```python
from build123d import *

# Parameters (mm, degrees)
SKETCH1_W           = 60
SKETCH1_H           = 60
BOSS_EXTRUDE1_DEPTH = 6
SKETCH2_R           = 1.15
CUT_EXTRUDE1_DEPTH  = 43.848570571
SKETCH3_R           = 1.15
CUT_EXTRUDE2_DEPTH  = 4
CUT_EXTRUDE3_DEPTH  = 3
SKETCH5_R           = 1.15
CUT_EXTRUDE4_DEPTH  = 43.532340636


with BuildPart() as part:
    # Sketch1 → Boss-Extrude1 (new body)
    with BuildSketch(Plane.XY):
        Rectangle(SKETCH1_W, SKETCH1_H)
    extrude(amount=BOSS_EXTRUDE1_DEPTH)

    # Sketch2 → Cut-Extrude1 (cut, through all)
    with BuildSketch(Plane.XY.offset(6)):
        with BuildLine():
            ThreePointArc((-25, 26.15), (-26.15, 25), (-25, 23.85))
            Line((-25, 23.85), (-25, 26.15))
        make_face()
        with BuildLine():
            Line((-25, 26.15), (-25, 23.85))
            ThreePointArc((-25, 23.85), (-24.186827202, 24.186827202), (-23.85, 25))
            ThreePointArc((-23.85, 25), (-24.186827202, 25.813172798), (-25, 26.15))
        make_face()
        with Locations((25, 25)):
            Circle(SKETCH2_R)
        with Locations((25, -25)):
            Circle(SKETCH2_R)
        with Locations((-25, -25)):
            Circle(SKETCH2_R)
    extrude(amount=-CUT_EXTRUDE1_DEPTH, mode=Mode.SUBTRACT)

    # Sketch3 → Cut-Extrude2 (cut)
    # profile 1 of 4: a face of its own
    with BuildSketch(Plane.XY.offset(6)):
        Polygon((-26.212435565, 22.9), (-23.787564435, 22.9), (-22.575128869, 25), (-23.787564435, 27.1), (-26.212435565, 27.1), (-27.424871131, 25), align=None)
        with Locations((-25, 25)):
            Circle(SKETCH3_R, mode=Mode.SUBTRACT)
    # profile 2 of 4: a face of its own
    with BuildSketch(Plane.XY.offset(6)):
        Polygon((22.575128869, 25), (23.787564435, 27.1), (26.212435565, 27.1), (27.424871131, 25), (26.212435565, 22.9), (23.787564435, 22.9), align=None)
        with Locations((25, 25)):
            Circle(SKETCH3_R, mode=Mode.SUBTRACT)
    # profile 3 of 4: a face of its own
    with BuildSketch(Plane.XY.offset(6)):
        Polygon((26.212435565, -22.9), (23.787564435, -22.9), (22.575128869, -25), (23.787564435, -27.1), (26.212435565, -27.1), (27.424871131, -25), align=None)
        with Locations((25, -25)):
            Circle(SKETCH3_R, mode=Mode.SUBTRACT)
    # profile 4 of 4: a face of its own
    with BuildSketch(Plane.XY.offset(6)):
        Polygon((-22.575128869, -25), (-23.787564435, -27.1), (-26.212435565, -27.1), (-27.424871131, -25), (-26.212435565, -22.9), (-23.787564435, -22.9), align=None)
        with Locations((-25, -25)):
            Circle(SKETCH3_R, mode=Mode.SUBTRACT)
    extrude(amount=-CUT_EXTRUDE2_DEPTH, mode=Mode.SUBTRACT)

    # Sketch4 → Cut-Extrude3 (cut)
    with BuildSketch(Plane(origin=(0, 0, 0), x_dir=(-1, 0, 0), z_dir=(0, 0, -1))):
        with BuildLine():
            ThreePointArc((-4, 3.9), (-2.51507576, 4.51507576), (-1.9, 6))
            Line((-1.9, 6), (-4, 6))
            Line((-4, 6), (-4, 3.9))
        make_face()
        with BuildLine():
            Line((-4, 6), (-1.9, 6))
            ThreePointArc((-1.9, 6), (-5.48492424, 7.48492424), (-4, 3.9))
            Line((-4, 3.9), (-4, 6))
        make_face()
        with BuildLine():
            ThreePointArc((6.1, 6), (4, 8.1), (1.9, 6))
            Line((1.9, 6), (4, 6))
            Line((4, 6), (4, 3.9))
            ThreePointArc((4, 3.9), (5.48492424, 4.51507576), (6.1, 6))
        make_face()
        with BuildLine():
            Line((4, 6), (1.9, 6))
            ThreePointArc((1.9, 6), (2.51507576, 4.51507576), (4, 3.9))
            Line((4, 3.9), (4, 6))
        make_face()
        with BuildLine():
            ThreePointArc((4, -3.9), (2.51507576, -4.51507576), (1.9, -6))
            Line((1.9, -6), (4, -6))
            Line((4, -6), (4, -3.9))
        make_face()
        with BuildLine():
            Line((4, -6), (1.9, -6))
            ThreePointArc((1.9, -6), (4, -8.1), (6.1, -6))
            ThreePointArc((6.1, -6), (5.48492424, -4.51507576), (4, -3.9))
            Line((4, -3.9), (4, -6))
        make_face()
        with BuildLine():
            ThreePointArc((-4, -3.9), (-5.48492424, -7.48492424), (-1.9, -6))
            Line((-1.9, -6), (-4, -6))
            Line((-4, -6), (-4, -3.9))
        make_face()
        with BuildLine():
            Line((-4, -6), (-1.9, -6))
            ThreePointArc((-1.9, -6), (-2.51507576, -4.51507576), (-4, -3.9))
            Line((-4, -3.9), (-4, -6))
        make_face()
    extrude(amount=-CUT_EXTRUDE3_DEPTH, mode=Mode.SUBTRACT)

    # Sketch5 → Cut-Extrude4 (cut, through all)
    with BuildSketch(Plane(origin=(0, 0, 3), x_dir=(-1, 0, 0), z_dir=(0, 0, -1))):
        with Locations((-4, 6)):
            Circle(SKETCH5_R)
        with Locations((4, 6)):
            Circle(SKETCH5_R)
        with Locations((4, -6)):
            Circle(SKETCH5_R)
        with Locations((-4, -6)):
            Circle(SKETCH5_R)
    extrude(amount=-CUT_EXTRUDE4_DEPTH, mode=Mode.SUBTRACT)


solid = part.part
```
Geometry: final body of the model. Coordinates: model frame, mm. A direction names the side the tool comes from. Coordinates: 2 decimals unless noted, no trailing zeros. Order: outer loops, then holes, each group sorted by start corner. A loop starts at its lowest first (then second) coordinate and runs counter-clockwise, first axis right, second up. Notation, with made-up numbers: (54.25, -3.5) - (108.25, -3.5) arc R23 ccw to (108.25, 18.5) - close; hole circle Ø9 at (83, 86). An arc over 180 degrees is marked (long way). Return JSON: item names as keys, results as strings. Group by question number.
1. Pull-direction query (Y, two-part tool) for faces 1 (the face through (-23.173, 26.035, 4.028)), 2 (the face through (0, -30, 3)), 3 (the face through (30, 0, 3)); classes: pulls with the +Y half, pulls with the -Y half, needs draft (parallel to the pull), parting line crosses it, or undercut.
2. Cut plane B-B (z = 4.5). Count the separate pieces of the cut face and the enclosed holes in it, plus the area to 3 significant figures.
3. Set-up query: faces 4 (the face through (-26.81, -26.065, 4.028)), 5 (the face through (4.15, -4.86, 4.48)), 6 (the face through (-5, 5, 3)). Return all of +Z, -Z, +X, -X, +Y, -Y with unobstructed straight access to the full face (end or side cutting, diameter ignored); none if empty.
4. Material intervals for line 1 along Y through (x, z) = (4, 1.45); line 2 along Y through (x, z) = (25, 0.6); line 3 along X through (y, z) = (-6, 0.75), sorted ascending. Write a range as [from, to].
5. Pin query (flat end, axial travel): pin 1 (3.5 mm diameter, centred on x = 25, y = 24.5, fed in from +Z); pin 2 (1.3 mm diameter, centred on x = 5, y = 6.5, fed in from -Z); pin 3 (3.5 mm diameter, centred on x = -25, y = -25, fed in from +Z). Return the tip coordinate at first contact, or that it passes through.
6. Cut plane A-A (x = 25). Output: boundary loops of the cut face in (y, z), plus the area to 3 significant figures.
Resolved:
{
 "1": {"face 1": "undercut", "face 2": "pulls with the -Y half", "face 3": "needs draft"},
 "2": {"separate pieces": "1", "enclosed holes": "8", "area": "3,520 mm²"},
 "3": {"face 4": "+Z", "face 5": "+Z, -Z", "face 6": "-Z"},
 "4": {"line 1": "y = [-30, -8.1], [-3.9, 3.9], [8.1, 30]", "line 2": "y = [-30, -26.15], [-23.85, 23.85], [26.15, 30]", "line 3": "x = [-30, -6.1], [-1.9, 1.9], [6.1, 30]"},
 "5": {"pin 1": "stops at z = 6", "pin 2": "stops at z = 3", "pin 3": "stops at z = 2"},
 "6": {"outline": "(-30, 0) - (-26.15, 0) - (-26.15, 2) - (-27.1, 2) - (-27.1, 6) - (-30, 6) - close; (-23.85, 0) - (23.85, 0) - (23.85, 2) - (22.9, 2) - (22.9, 6) - (-22.9, 6) - (-22.9, 2) - (-23.85, 2) - close; (26.15, 0) - (30, 0) - (30, 6) - (27.1, 6) - (27.1, 2) - (26.15, 2) - close", "area": "317 mm²"}
}
